Work out the finished part from the listing and answer in its coordinate system (mm). Coordinates: 2 decimals unless noted, no trailing zeros. Loops run counter-clockwise (first coordinate to the right, second up) from the corner with the lowest first, then second, coordinate; pieces in that order, holes last.
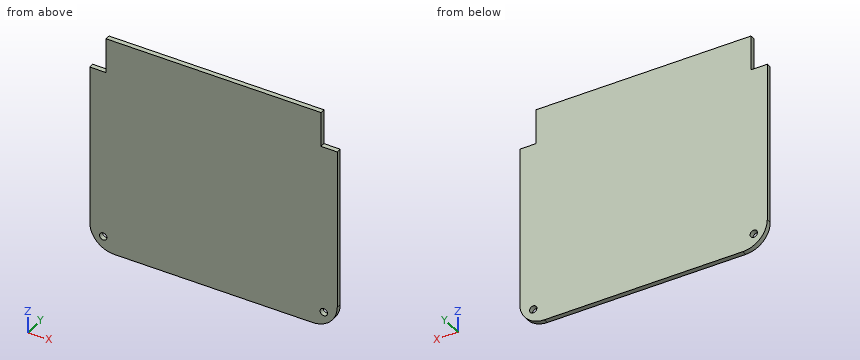
```python
from build123d import *

# Parameters (mm, degrees)
EXTRUDE_1_DEPTH     = 2
SKETCH_3_R          = 1.5
CUT_EXTRUDE_1_DEPTH = 10


with BuildPart() as part:
    # 草图1 → 凸台-拉伸1 (new body)
    with BuildSketch(Plane(origin=(0, 0, 0), x_dir=(1, 0, 0), z_dir=(0, 1, 0))):
        with BuildLine():
            Line((0, -100.302122976), (0, -86.002122976))
            Line((0, -86.002122976), (6.65, -86.002122976))
            Line((6.65, -86.002122976), (6.65, -20.302122976))
            ThreePointArc((6.65, -20.302122976), (3.721067812, -13.231055164), (-3.35, -10.302122976))
            Line((-3.35, -10.302122976), (-84.35, -10.302122976))
            ThreePointArc((-84.35, -10.302122976), (-91.421067812, -13.231055164), (-94.35, -20.302122976))
            Line((-94.35, -20.302122976), (-94.35, -86.002122976))
            Line((-94.35, -86.002122976), (-87.7, -86.002122976))
            Line((-87.7, -86.002122976), (-87.7, -100.302122976))
            Line((-87.7, -100.302122976), (0, -100.302122976))
        make_face()
    extrude(amount=EXTRUDE_1_DEPTH)

    # 草图3 → 切除-拉伸1 (cut)
    with BuildSketch(Plane(origin=(0, 2, 0), x_dir=(1, 0, 0), z_dir=(0, 1, 0))):
        with Locations(Location((-88.85, -16.302122976, 0), (0, 0, 270))):
            Circle(SKETCH_3_R)
        with Locations(Location((1.15, -16.302122976, 0), (0, 0, 270))):
            Circle(SKETCH_3_R)
    extrude(amount=-CUT_EXTRUDE_1_DEPTH, mode=Mode.SUBTRACT)


solid = part.part
```
1. Straight lines are drawn through the part: probe 1 along Z at (x, y) = (1.5, 1.25); probe 2 along Z at (x, y) = (-88.85, 0.4); probe 3 along X at (y, z) = (1.55, 94). For each, find the intervals that lie inside material, in ascending order.
2. A cutting plane is placed at B-B, the plane x = 1.15. Give the vertices of the cut face in (y, z).
3. Each of these flat-tipped pins is pushed along its axis until it touches: P1, Ø0.6, axis at y = 1.5, z = 91, coming from the -X side; P2, Ø1, axis at x = -91, y = 1.5, coming from the +Z side; P3, Ø0.6, axis at y = 1, z = 91, coming from the +X side. Where does it stop, or does it pass through?
4. A cutting plane is placed at A-A, the plane y = 0.85. Give the vertices of the cut face in (x, z), then the cut area to 3 significant figures.
Answers below:
1. probe 1: z = 11.56 to 14.84, 17.76 to 86
1. probe 2: z = 11.37 to 14.8, 17.8 to 86
1. probe 3: x = -87.7 to 0
2. outline: (0, 11.37) - (2, 11.37) - (2, 14.8) - (0, 14.8) - close; (0, 17.8) - (2, 17.8) - (2, 86) - (0, 86) - close
3. P1: stops at x = -87.7
3. P2: stops at z = 86
3. P3: stops at x = 0
4. outline: (-94.35, 20.3) arc R10 ccw to (-84.35, 10.3) - (-3.35, 10.3) arc R10 ccw to (6.65, 20.3) - (6.65, 86) - (0, 86) - (0, 100.3) - (-87.7, 100.3) - (-87.7, 86) - (-94.35, 86) - close; hole circle Ø3 at (-88.85, 16.3); hole circle Ø3 at (1.15, 16.3)
4. area: 8,840 mm2
